Autodesk Inventor part; units mm, degrees
ref_plane "YZ Plane" through (0, 0, 0) normal (1, 0, 0) x (0, 1, 0)
ref_plane "XZ Plane" through (0, 0, 0) normal (0, 1, 0) x (-1, 0, 0)
ref_plane "XY Plane" through (0, 0, 0) normal (0, 0, 1) x (1, 0, 0)
sketch "Sketch1" plane through (0, 0, 0) normal (0, 1, 0) x (-1, 0, 0)
  line L0 (75, -40) -> (-75, -40)
  line L1 (-75, -40) -> (-75, 40)
  line L2 (-75, 40) -> (75, 40)
  line L3 (75, 40) -> (75, -40)
  line L4 (75, -40) -> (-75, 40) construction
  line L5 (-75, -40) -> (75, 40) construction
  point P0 (0, 0)
  dimension "d0" = 80
  dimension "d1" = 150
extrude "Extrusion1" add sketch "Sketch1" along normal blind 80
sketch "Sketch2" plane through (75, 0, 40) normal (1, 0, 0) x (0, 0, -1)
  line L0 (0, 0) -> (0, 80)
  line L1 (0, 40) -> (80, 40)
  line L2 (80, 0) -> (80, 80)
  line L3 (40, 0) -> (40, 80)
  line L4 (0, 80) -> (80, 80)
  line L5 (75, 72.5) -> (5, 72.5)
  line L6 (5, 72.5) -> (5, 7.5)
  line L7 (5, 7.5) -> (75, 7.5)
  line L8 (75, 7.5) -> (75, 72.5)
  line L9 (75, 72.5) -> (5, 7.5) construction
  line L10 (5, 72.5) -> (75, 7.5) construction
  point P0 (40, 40)
  dimension "d4" = 70
  dimension "d5" = 65
extrude "Extrusion2" cut sketch "Sketch2" against normal blind 143.6625 contours L6 L5 L3 L1 | L1 L3 L7 L6 | L3 L5 L8 L1 | L1 L8 L7 L3
sketch "Sketch8" plane through (-75, 0, 40) normal (0, 0, 1) x (1, 0, 0)
  line L0 (0, 0) -> (0, 80)
  line L1 (0, 40) -> (75, 40) construction
  line L2 (75, 40) -> (75, 0) construction
  line L3 (0, 20) -> (75, 20) construction
  circle A0 centre (75, 20) radius 5
  dimension "d24" = 10
extrude "Extrusion5" add sketch "Sketch8" along normal blind 25
sketch "Sketch9" plane through (75, 0, -40) normal (0, 0, -1) x (-1, 0, 0)
  line L0 (0, 0) -> (0, 80)
  line L1 (0, 40) -> (75, 40) construction
  line L2 (75, 40) -> (75, 0) construction
  circle A0 centre (75, 20) radius 5
  line L3 (0, 20) -> (75, 20) construction
  circle A1 centre (75, 20) radius 5
  dimension "d25" = 10
extrude "Extrusion6" add sketch "Sketch9" along normal blind 25
fillet "Fillet1" radius 4.7625 1 edges at (-5, 20, 65)
fillet "Fillet2" radius 4.7625 1 edges at (5, 20, -65)
fillet "Fillet3" radius 4.7625 10 edges at (-75, 40, -40) (-75, 40, 40) (75, 40, 40) (75, 40, -40) (-75, 80, 0) (75, 80, 0) (-75, 0, 0) (0, 0, -40) (75, 0, 0) (0, 0, 40)
sketch "Sketch10" plane through (0, 80, 0) normal (0, 1, 0) x (1, 0, 0)
  line L0 (50, 35) -> (-50, 35)
  line L1 (-50, 35) -> (-50, -35)
  line L2 (-50, -35) -> (50, -35)
  line L3 (50, -35) -> (50, 35)
  line L4 (50, 35) -> (-50, -35) construction
  line L5 (-50, 35) -> (50, -35) construction
  line L6 (40, 25) -> (-40, 25)
  line L7 (-40, 25) -> (-40, -25)
  line L8 (-40, -25) -> (40, -25)
  line L9 (40, -25) -> (40, 25)
  line L10 (40, 25) -> (-40, -25) construction
  line L11 (-40, 25) -> (40, -25) construction
  point P0 (0, 0)
  dimension "d29" = 70
  dimension "d30" = 100
  dimension "d31" = 10
  dimension "d32" = 10
extrude "Extrusion7" add sketch "Sketch10" along normal blind 10
sketch "Sketch11" plane through (0, 90, 0) normal (0, 1, 0) x (1, 0, 0)
  line L0 (75.0062, 40.005) -> (-75.0062, 40.005)
  line L1 (-75.0062, 40.005) -> (-75.0062, -40.005)
  line L2 (-75.0062, -40.005) -> (75.0062, -40.005)
  line L3 (75.0062, -40.005) -> (75.0062, 40.005)
  line L4 (75.0062, 40.005) -> (-75.0062, -40.005) construction
  line L5 (-75.0062, 40.005) -> (75.0062, -40.005) construction
  point P0 (0, 0)
  dimension "d35" = 80.01
  dimension "d36" = 150.0124
extrude "Extrusion8" add sketch "Sketch11" along normal blind 10
sketch "Sketch12" plane through (-75.0062, 90, 40.005) normal (0, 0, 1) x (1, 0, 0)
  line L0 (150.0124, 10) -> (0, 10) construction
  line L1 (150.0124, 0) -> (0, 0) construction
  line L2 (0, 10) -> (150.0124, 0) construction
  line L3 (0, 0) -> (150.0124, 10) construction
  line L4 (35.0062, 0) -> (115.0062, 0)
  line L5 (110.0062, 10) -> (40.0062, 10)
  line L6 (40.0062, 10) -> (40.0062, 0)
  line L7 (40.0062, 0) -> (110.0062, 0)
  line L8 (110.0062, 0) -> (110.0062, 10)
  line L9 (110.0062, 10) -> (40.0062, 0) construction
  line L10 (40.0062, 10) -> (110.0062, 0) construction
  point P0 (75.0062, -90)
  point P1 (75.0062, 5)
  dimension "d39" = 70
extrude "Extrusion9" add sketch "Sketch12" along normal blind 10
sketch "Sketch13" plane through (75.0062, 90, -40.005) normal (0, 0, -1) x (-1, 0, 0)
  line L0 (0, 0) -> (150.0124, 0)
  line L1 (150.0124, 0) -> (150.0124, 10)
  line L2 (0, 10) -> (150.0124, 10)
  line L3 (0, 0) -> (0, 10)
  line L4 (0, 10) -> (150.0124, 0) construction
  line L5 (150.0124, 10) -> (0, 0) construction
  line L6 (35.0062, 0) -> (115.0062, 0)
  line L7 (110.0062, 10) -> (40.0062, 10)
  line L8 (40.0062, 10) -> (40.0062, 0)
  line L9 (40.0062, 0) -> (110.0062, 0)
  line L10 (110.0062, 0) -> (110.0062, 10)
  line L11 (110.0062, 10) -> (40.0062, 0) construction
  line L12 (40.0062, 10) -> (110.0062, 0) construction
  point P0 (75.0062, -90)
  point P1 (75.0062, 5)
  point P2 (110.0062, 10)
  point P3 (40.0062, 10)
  dimension "d42" = 70
extrude "Extrusion10" add sketch "Sketch13" along normal blind 10 contours L8 L2 L10 L0
fillet "Fillet4" radius 25.4 4 edges at (50, 85, -35) (50, 85, 35) (-50, 85, 35) (-50, 85, -35)
properties part number "Battery Container" material "Iron, Malleable"
Can you work these out from the model? Positions are in its coordinate system, mm. A direction names the side the tool comes from. Coordinates: 2 decimals unless noted, no trailing zeros. Loops run counter-clockwise (first coordinate to the right, second up) from the corner with the lowest first, then second, coordinate; pieces in that order, holes last.
Item 1: I'm going to push flat-ended pins straight in: pin 1 (3 mm diameter, centred on x = -58.5, y = 95, fed in from +Z) (3 decimals); pin 2 (8 mm diameter, centred on y = 83.5, z = -9.5, fed in from +X); pin 3 (6 mm diameter, centred on y = 22.5, z = -7.5, fed in from -X); pin 4 (6 mm diameter, centred on y = 86, z = 40, fed in from +X). Where does each tip first touch, or does it pass through?
Answers below:
pin 1: stops at z = 40.005
pin 2: stops at x = 72.36
pin 3: stops at x = -75
pin 4: passes through
Item 2: Suppose I cut it at A-A (z = 6). Please give me the cut outline in (x, y) (1 decimal), then the cut area to 3 significant figures.
Answers below:
outline: (-75, 4.8) arc R4.8 ccw to (-70.2, 0) - (70.2, 0) arc R4.8 ccw to (75, 4.8) - (75, 7.5) - (-68.7, 7.5) - (-68.7, 72.5) - (75, 72.5) - (75, 75.2) arc R4.8 ccw to (70.2, 80) - (50, 80) - (50, 90) - (75, 90) - (75, 100) - (-75, 100) - (-75, 90) - (-50, 90) - (-50, 80) - (-70.2, 80) arc R4.8 ccw to (-75, 75.2) - close; hole (-40, 80) - (40, 80) - (40, 90) - (-40, 90) - close
area: 4,340 mm2
Item 3: Suppose I cut it at D-D (y = 87). Please give me the cut outline in (x, z).
Answers below:
outline: (-50, -9.6) arc R25.4 ccw to (-24.6, -35) - (24.6, -35) arc R25.4 ccw to (50, -9.6) - (50, 9.6) arc R25.4 ccw to (24.6, 35) - (-24.6, 35) arc R25.4 ccw to (-50, 9.6) - close; hole (-40, -25) - (40, -25) - (40, 25) - (-40, 25) - close
Item 4: Which directions (+Z, -Z, +X, -X, +Y, -Y) give clear straight access to the entire face, cutting with the end or side of a thin tool? Please do faces 4 (the face through (35, 95, -45)), 5 (the face through (1.08, 24.88, -49.98)), 6 (the face through (4, 72.5, 0)), 7 (the face through (50, 85, 0)), 8 (the face through (-1, 90, -45)).
Answers below:
face 4: -Z, +X, +Y, -Y
face 5: -Z
face 6: +X
face 7: +Z, -Z, +X
face 8: none
Item 5: If we mould it in two halves opening along Z, with no side actions, what happens to faces 1 (the face through (-73.64, 78.57, -0.56)), 2 (the face through (4, 7.5, 0)), 3 (the face through (55, 95, 40.005))? For each: released by +Z, released by -Z, zero draft, split by the parting line, or undercut.
Answers below:
face 1: zero draft
face 2: undercut
face 3: released by +Z
Item 6: Suppose I cut it at B-B (z = 38). Please give me the cut outline in (x, y) (1 decimal), then the cut area to 3 significant figures.
Answers below:
outline: (-75, 90) - (75, 90) - (75, 100) - (-75, 100) - close; (-74.1, 4.8) arc R3.9 ccw to (-70.2, 0.9) - (70.2, 0.9) arc R3.9 ccw to (74.1, 4.8) - (74.1, 78) arc R4.8 ccw to (70.2, 80) - (-70.2, 80) arc R4.8 ccw to (-74.1, 78) - close
area: 13,200 mm2
Item 7: Please list where these lines run through material, in increasing order: L1, parallel to Y at x = 20, z = 1; L2, parallel to Z at x = -44, y = 60; L3, parallel to Y at x = 48, z = 18.5.
Answers below:
L1: y = 0 to 7.5, 72.5 to 80, 90 to 100
L2: z = -40 to -35, 35 to 40
L3: y = 0 to 7.5, 72.5 to 100
